Drawing for the job (mm, zero at the part's lowest x, y, z). Give positions to 0.01 mm unless a question says otherwise; leave off trailing zeros. Loops run counter-clockwise (first coordinate to the right, second up) from the corner with the lowest first, then second, coordinate; pieces in that order, holes last. Notation, with made-up numbers: (-18, -37.5) -> (32, -37.5) arc R16 ccw to (32, -17.5) -> close; hole circle Ø5 at (50, -33). An arc over 180 degrees is marked (long way). Write item = value, one per line.
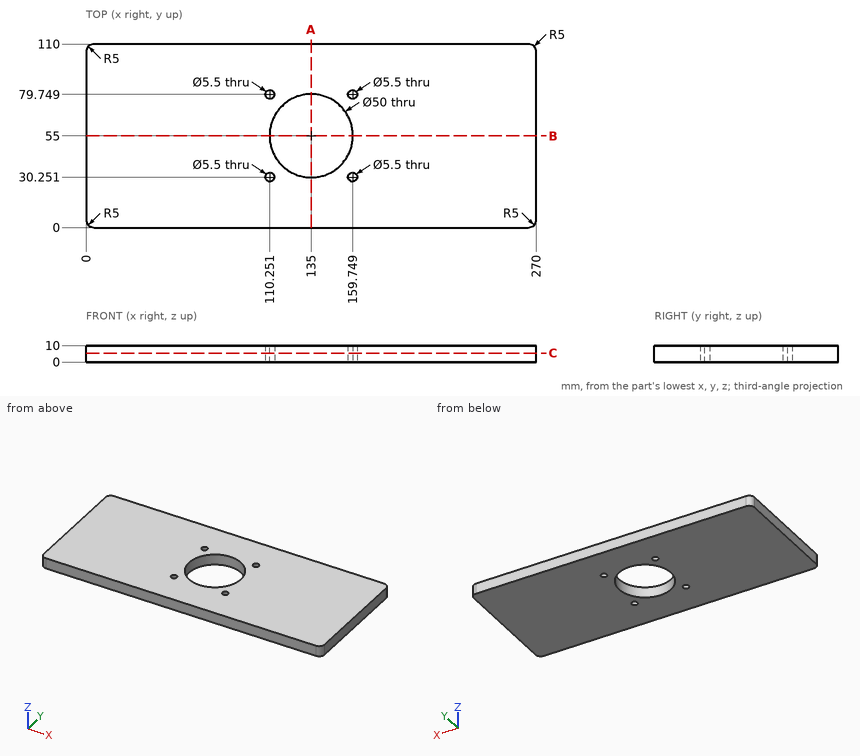
1) Slice it at C-C, the plane z = 5.5. List the corners of the cut face in (x, y).
Resolved:
outline = (0, 5) arc R5 ccw to (5, 0) -> (265, 0) arc R5 ccw to (270, 5) -> (270, 105) arc R5 ccw to (265, 110) -> (5, 110) arc R5 ccw to (0, 105) -> close; hole circle Ø5.5 at (110.25, 30.25); hole circle Ø5.5 at (110.25, 79.75); hole circle Ø50 at (135, 55); hole circle Ø5.5 at (159.75, 30.25); hole circle Ø5.5 at (159.75, 79.75)
2) Drill centre lines: line 1 along X through (y, z) = (81, 3); line 2 along X through (y, z) = (70.5, 3.5) (1 decimal); line 3 along X through (y, z) = (75.5, 4.5). Where is each one in solid material? Low to high. Write a range as [from, to].
Resolved:
line_1 = [0, 107.8], [112.7, 157.3], [162.2, 270]
line_2 = [0, 115.4], [154.6, 270]
line_3 = [0, 120.69], [149.31, 270]
3) Slice it at A-A, the plane x = 135. List the corners of the cut face in (y, z).
Resolved:
outline = (0, 0) -> (30, 0) -> (30, 10) -> (0, 10) -> close; (80, 0) -> (110, 0) -> (110, 10) -> (80, 10) -> close
4) Slice it at B-B, the plane y = 55. List the corners of the cut face in (x, z).
Resolved:
outline = (0, 0) -> (110, 0) -> (110, 10) -> (0, 10) -> close; (160, 0) -> (270, 0) -> (270, 10) -> (160, 10) -> close
5) Drop a flat-ended pin along its axis: P1, Ø4.5, axis at x = 159.75, y = 79.75, coming from the -Z side. Give the stop position or say it passes through.
Resolved:
P1 = through
